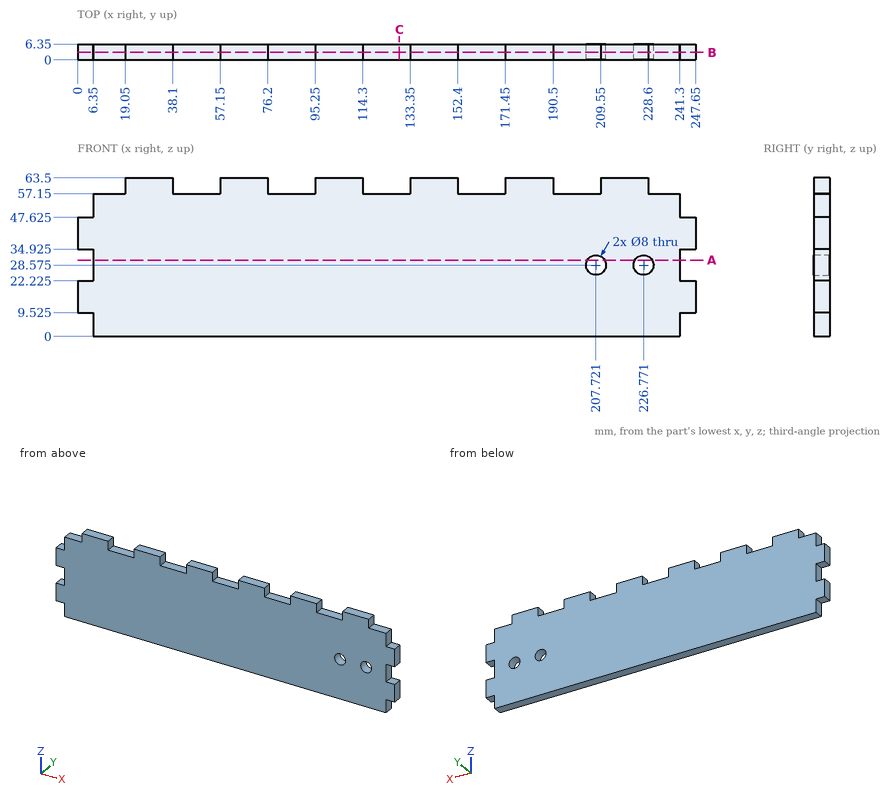
Can you work these out from the drawing? Everything is in mm from the part's minimum corner. Round coordinates to 2 decimals unless told otherwise and drop trailing zeros. Order: outer loops, then holes, each group sorted by start corner. A loop starts at its lowest first (then second) coordinate and runs counter-clockwise, first axis right, second up. Notation, with made-up numbers: (20, -12) - (59, -12) arc R33 cw to (59, 23) - close; hole circle Ø6 at (19, 40.25). An arc over 180 degrees is marked (long way). Answer in a Markdown table with one row per item.
(1) Please list where these lines run through material, in increasing order: L1, parallel to Z at x = 196, y = 3; L2, parallel to X at y = 5.25, z = 52.5; L3, parallel to Z at x = 228.5, y = 2.5. Write a range as from..to.
From the geometry:
| item | result |
|---|---|
| L1 | z = 0..57.15 |
| L2 | x = 6.35..241.3 |
| L3 | z = 0..24.97, 32.18..63.5 |
(2) For P1, Ø3, axis at x = 237.5, y = 2.5, coming from the +Z side; P2, Ø3, axis at y = 4.5, z = 61.5, coming from the +X side; P3, Ø3, axis at x = 2, y = 2.5, coming from the -Z side (3 decimals); P4, Ø6.5, axis at x = 226.77, z = 28.58, coming from the -Y side, each with a flat end and sliding along its axis, tell me the tip position at first contact or that it passes through.
From the geometry:
| item | result |
|---|---|
| P1 | stops at z = 57.15 |
| P2 | stops at x = 228.6 |
| P3 | stops at z = 9.525 |
| P4 | passes through |
(3) Suppose I cut it at B-B, the plane y = 3. Count the separate pieces of the cut face and the enclosed holes in it, plus the area to 3 significant figures.
From the geometry:
| item | result |
|---|---|
| separate pieces | 1 |
| enclosed holes | 2 |
| area | 14,400 mm2 |
(4) Suppose I cut it at A-A, the plane z = 30.5. Please give me the cut outline in (x, y).
From the geometry:
| item | result |
|---|---|
| outline | (6.35, 0) - (204.21, 0) - (204.21, 6.35) - (6.35, 6.35) - close; (211.23, 0) - (223.26, 0) - (223.26, 6.35) - (211.23, 6.35) - close; (230.28, 0) - (241.3, 0) - (241.3, 6.35) - (230.28, 6.35) - close |
(5) Suppose I cut it at C-C, the plane x = 129. Please give me the cut outline in (y, z).
From the geometry:
| item | result |
|---|---|
| outline | (0, 0) - (6.35, 0) - (6.35, 57.15) - (0, 57.15) - close |
